Could you check a few things on this model? Use its own coordinates, in mm. A direction names the side the tool comes from. Round coordinates to 2 decimals unless told otherwise and drop trailing zeros. Order: outer loops, then holes, each group sorted by start corner. A loop starts at its lowest first (then second) coordinate and runs counter-clockwise, first axis right, second up. Notation, with made-up numbers: (2, 4.25) - (23, 4.25) arc R14 ccw to (23, 20.25) - close; hole circle Ø8 at (34.5, -17). An arc over 180 degrees is marked (long way). Use one line per item in the form item = value.
from build123d import *

# Parameters (mm, degrees)
SKETCH042_W           = 13.85
SKETCH042_H           = 13.85
PAD020_DEPTH          = 10
POCKET016_DEPTH       = 8.2
SKETCH054_R           = 4.5
POCKET025_DEPTH       = 0.001
POCKET025_DEPTH_BACK  = 10.001
SKETCH044_W           = 12.45
SKETCH044_H           = 12.45
POCKET017_DEPTH       = 0.85
SKETCH045_W           = 3.65
SKETCH045_H           = 2
POCKET018_DEPTH       = 2
POLARPATTERN004_COUNT = 4
POCKET019_DEPTH       = 6.926
POCKET020_DEPTH       = 6.926
POCKET021_DEPTH       = 6.926
POCKET022_DEPTH       = 6.926
SKETCH050_R           = 0.75
HOLE_DEPTH            = 6
SKETCH052_W           = 2
SKETCH052_H           = 2.1
SKETCH052_W_2         = 2.1
SKETCH052_H_2         = 2
POCKET023_DEPTH       = 3
SKETCH053_W           = 1
SKETCH053_H           = 2.1
SKETCH053_W_2         = 2.1
SKETCH053_H_2         = 1
POCKET024_DEPTH       = 5.851
FILLET_R              = 0.5
CHAMFER001_1_SIZE2    = 0.5
CHAMFER001_1_SIZE     = 0.8
CHAMFER001_2_SIZE2    = 0.5
CHAMFER001_2_SIZE     = 0.8


with BuildPart() as part:
    # Sketch042 → Pad020 (new body)
    with BuildSketch(Plane.XY):
        Rectangle(SKETCH042_W, SKETCH042_H)
    extrude(amount=PAD020_DEPTH)

    # Sketch043 → Pocket016 (cut)
    with BuildSketch(Plane.XY):
        with BuildLine():
            Line((-5.725, 4.025), (-5.725, -5.725))
            Line((-5.725, -5.725), (4.025, -5.725))
            ThreePointArc((5.725, -4.025), (4.305761, -4.305761), (4.025, -5.725))
            Line((5.725, -4.025), (5.725, 5.725))
            Line((5.725, 5.725), (-4.025, 5.725))
            ThreePointArc((-5.725, 4.025), (-4.305761, 4.305761), (-4.025, 5.725))
        make_face()
    extrude(amount=POCKET016_DEPTH, mode=Mode.SUBTRACT)

    # Sketch054 → Pocket025 (cut, two sides)
    with BuildSketch(Plane.XY) as pocket025_sk:
        Circle(SKETCH054_R)
    extrude(amount=-POCKET025_DEPTH, mode=Mode.SUBTRACT)
    extrude(pocket025_sk.sketch, amount=POCKET025_DEPTH_BACK, mode=Mode.SUBTRACT)

    # Sketch055 → Groove003 (revolve, cut)
    with BuildSketch(Plane.XZ):
        Polygon((4.5, 9.9), (5.7, 8.2), (4.5, 8.2), align=None)
    revolve(axis=Axis((0, 0, 0), (0, 0, 1)), mode=Mode.SUBTRACT)

    # Sketch044 → Pocket017 (cut)
    with BuildSketch(Plane.XY):
        Rectangle(SKETCH044_W, SKETCH044_H)
    extrude(amount=POCKET017_DEPTH, mode=Mode.SUBTRACT)

    # Sketch045 → Pocket018 (cut)
    with BuildSketch(Plane.XY):
        with Locations((0, 5.925)):
            Rectangle(SKETCH045_W, SKETCH045_H)
    pocket018 = extrude(amount=POCKET018_DEPTH, mode=Mode.SUBTRACT)

    # PolarPattern004: Pocket018 ×4 about axis
    polarpattern004_axis = Axis((0, 0, 0), (0, 0, 1))
    for i in range(1, POLARPATTERN004_COUNT):
        add(pocket018.rotate(polarpattern004_axis, i * 360 / POLARPATTERN004_COUNT), mode=Mode.SUBTRACT)

    # Sketch046 → Pocket019 (cut, through all)
    with BuildSketch(Plane.XZ):
        with BuildLine():
            ThreePointArc((1.6, 5.9), (0, 7.5), (-1.6, 5.9))
            Line((-1.6, 5.9), (-1.6, 1.9))
            Line((-1.6, 1.9), (-1.825, 1.9))
            Line((-1.825, 1.9), (-1.825, -0.1))
            Line((1.825, -0.1), (-1.825, -0.1))
            Line((1.825, 1.9), (1.825, -0.1))
            Line((1.6, 1.9), (1.825, 1.9))
            Line((1.6, 5.9), (1.6, 1.9))
        make_face()
    extrude(amount=-POCKET019_DEPTH, mode=Mode.SUBTRACT)

    # Sketch047 → Pocket020 (cut, through all)
    with BuildSketch(Plane.XZ):
        with BuildLine():
            ThreePointArc((1.325, 5.9), (0, 7.225), (-1.325, 5.9))
            Line((-1.325, 5.9), (-1.325, 1.9))
            Line((-1.325, 1.9), (-1.825, 1.9))
            Line((-1.825, 1.9), (-1.825, -0.1))
            Line((1.825, -0.1), (-1.825, -0.1))
            Line((1.825, 1.9), (1.825, -0.1))
            Line((1.325, 1.9), (1.825, 1.9))
            Line((1.325, 5.9), (1.325, 1.9))
        make_face()
    extrude(amount=POCKET020_DEPTH, mode=Mode.SUBTRACT)

    # Sketch048 → Pocket021 (cut, through all)
    with BuildSketch(Plane.YZ):
        with BuildLine():
            ThreePointArc((1.325, 5.9), (0, 7.225), (-1.325, 5.9))
            Line((-1.325, 5.9), (-1.325, 1.9))
            Line((-1.325, 1.9), (-1.825, 1.9))
            Line((-1.825, 1.9), (-1.825, -0.1))
            Line((1.825, -0.1), (-1.825, -0.1))
            Line((1.825, 1.9), (1.825, -0.1))
            Line((1.325, 1.9), (1.825, 1.9))
            Line((1.325, 5.9), (1.325, 1.9))
        make_face()
    extrude(amount=POCKET021_DEPTH, mode=Mode.SUBTRACT)

    # Sketch049 → Pocket022 (cut, through all)
    with BuildSketch(Plane.YZ):
        with BuildLine():
            ThreePointArc((1.325, 5.9), (0, 7.225), (-1.325, 5.9))
            Line((-1.325, 5.9), (-1.325, 2))
            Line((-1.325, 2), (-1.825, 2))
            Line((-1.825, 2), (-1.825, 0))
            Line((1.825, 0), (-1.825, 0))
            Line((1.825, 2), (1.825, 0))
            Line((1.325, 2), (1.825, 2))
            Line((1.325, 5.9), (1.325, 2))
        make_face()
    extrude(amount=-POCKET022_DEPTH, mode=Mode.SUBTRACT)

    # Sketch050 → Hole (cut)
    with BuildSketch(Plane.XY):
        with Locations((-5.225, 5.225)):
            Circle(SKETCH050_R)
        with Locations((5.225, -5.225)):
            Circle(SKETCH050_R)
    extrude(amount=HOLE_DEPTH, mode=Mode.SUBTRACT)

    # Sketch052 → Pocket023 (cut)
    with BuildSketch(Plane.XY):
        with Locations((-5.25, -4.2)):
            Rectangle(SKETCH052_W, SKETCH052_H)
        with Locations((4.2, 5.25)):
            Rectangle(SKETCH052_W_2, SKETCH052_H_2)
    extrude(amount=POCKET023_DEPTH, mode=Mode.SUBTRACT)

    # Sketch053 → Pocket024 (cut, through all)
    with BuildSketch(Plane.XY.offset(4.15)):
        with Locations((-5.75, -4.2)):
            Rectangle(SKETCH053_W, SKETCH053_H)
        with Locations((4.2, 5.75)):
            Rectangle(SKETCH053_W_2, SKETCH053_H_2)
    extrude(amount=POCKET024_DEPTH, mode=Mode.SUBTRACT)

    # Fillet
    fillet_edges = [part.edges().sort_by_distance(p)[0] for p in [
        (-6.925, 6.925, 5),
        (-6.925, -6.925, 5),
        (6.925, -6.925, 5),
        (6.925, 6.925, 5),
    ]]
    fillet(fillet_edges, radius=FILLET_R)

    # Chamfer001 1
    chamfer001_1_edges = [part.edges().sort_by_distance(p)[0] for p in [
        (-5.725, -4.2, 3),
    ]]
    chamfer001_1_side = part.faces().sort_by_distance((-5.725, 2.925, 0.9721))[0]
    chamfer(chamfer001_1_edges, length=CHAMFER001_1_SIZE, length2=CHAMFER001_1_SIZE2, reference=chamfer001_1_side)

    # Chamfer001 2
    chamfer001_2_edges = [part.edges().sort_by_distance(p)[0] for p in [
        (4.2, 5.725, 3),
    ]]
    chamfer001_2_side = part.faces().sort_by_distance((5.4875, 5.725, 0.9721))[0]
    chamfer(chamfer001_2_edges, length=CHAMFER001_2_SIZE, length2=CHAMFER001_2_SIZE2, reference=chamfer001_2_side)


with BuildPart() as part_1:
    # Body005 placement: moved
    add(part.part.moved(Location((0, 0, -5.9))))


solid = part_1.part
Item 1: I need wall thicknesses on L1, parallel to Y at x = 3, z = -2.25 (3 decimals); L2, parallel to X at y = -4, z = 3.25 (3 decimals). Which ranges of each line are inside material? Lowest first, please.
Found:
L1 = -6.925 to -5.725, 5.725 to 6.925
L2 = -6.925 to -6.25, -5.25 to -3.049, 3.049 to 6.925
Item 2: If we mould it in two halves opening along Y, with no side actions, what happens to faces 5 (the face through (-6, -5.25, 2)), 6 (the face through (1.825, -6.4, -4.7))? For each: released by +Y, released by -Y, zero draft, split by the parting line, or undercut.
Found:
face_5 = undercut
face_6 = zero draft
Item 3: Will these pins go through, and if not, where does the flat tip stop? P1, Ø2, axis at x = 5, y = -2, coming from the -Z side; P2, Ø5.5, axis at x = -2.5, y = -0.5, coming from the -Z side.
Found:
P1 = -5.05
P2 = 2.87
Item 4: For faces 1 (the face through (1.6, 6, -2)), 2 (the face through (-6.4, -1.825, -4.7)), 3 (the face through (-1.825, -6.4, -4.7)), 4 (the face through (-4.1, -6.225, -5.5)), which set-ups out of +Z, -Z, +X, -X, +Y, -Y let a thin tool reach every point of the face, with its end or its side?
Found:
face_1 = -Z, +Y
face_2 = -Z, +X, -X
face_3 = -Z, +Y, -Y
face_4 = -Z
Item 5: Imagine slicing it at C-C on z = 2.5. Please give me the cut outline in (x, y) (3 decimals), plus the area to 3 significant figures.
Found:
outline = (-6.925, -6.425) arc R0.5 ccw to (-6.425, -6.925) - (6.425, -6.925) arc R0.5 ccw to (6.925, -6.425) - (6.925, 6.425) arc R0.5 ccw to (6.425, 6.925) - (-6.425, 6.925) arc R0.5 ccw to (-6.925, 6.425) - close; hole (-6.25, -5.25) - (-5.25, -5.25) - (-5.25, -3.15) - (-6.25, -3.15) - close; hole circle Ø11.118 at (0, 0); hole (3.15, 5.25) - (5.25, 5.25) - (5.25, 6.25) - (3.15, 6.25) - close
area = 90.3 mm2
Item 6: Imagine slicing it at B-B on z = -1.5. State how many separate pieces and enclosed holes the cut face has, plus the area to 3 significant figures.
Found:
separate_pieces = 4
enclosed_holes = 2
area = 47.1 mm2
Item 7: Imagine slicing it at A-A on y = 0. Please give me the cut outline in (x, z) (3 decimals).
Found:
outline = (-6.925, 1.325) - (-5.725, 1.325) - (-5.725, 2.3) - (-5.7, 2.3) - (-4.5, 4) - (-4.5, 4.1) - (-6.925, 4.1) - close; (4.5, 4) - (5.7, 2.3) - (5.725, 2.3) - (5.725, 1.325) - (6.925, 1.325) - (6.925, 4.1) - (4.5, 4.1) - close
